The model under review builds one solid part; all positions refer to its coordinate system, in mm. A direction names the side the tool comes from. Coordinates: 2 decimals unless noted, no trailing zeros. Order: outer loops, then holes, each group sorted by start corner. A loop starts at its lowest first (then second) coordinate and runs counter-clockwise, first axis right, second up.
```python
from build123d import *

# Parameters (mm, degrees)
SKETCH2_W                    = 76
SKETCH2_H                    = 120
BASE_FLANGE1_DEPTH           = 1
EDGE_FLANGE1_STRIP_W         = 5.4732
EDGE_FLANGE1_STRIP_H         = 1
EDGE_FLANGE1_STRIP_CUT_DEPTH = 76
EDGE_FLANGE1_DEPTH           = 76
SKETCH10_R                   = 2.063994429
CUT_EXTRUDE1_DEPTH           = 1
SKETCH11_R                   = 5
SKETCH11_R_2                 = 17.5
CUT_EXTRUDE2_DEPTH           = 1


# Sheet-metal steps are written as plain solids
with BuildPart() as part:
    # Sketch2 → Base-Flange1 (new body)
    with BuildSketch(Plane.XY):
        Rectangle(SKETCH2_W, SKETCH2_H)
    extrude(amount=-BASE_FLANGE1_DEPTH)

    # Edge-Flange1 strip (across the edge) → Edge-Flange1 strip cut (cut)
    with BuildSketch(Plane(origin=(38, -60, -1), x_dir=(0, 1, 0), z_dir=(-1, 0, 0))):
        with Locations((-1, -0.5)):
            Rectangle(EDGE_FLANGE1_STRIP_W, EDGE_FLANGE1_STRIP_H)
    extrude(amount=EDGE_FLANGE1_STRIP_CUT_DEPTH, mode=Mode.SUBTRACT)

    # Edge-Flange1 section (across the edge) → Edge-Flange1 (add)
    with BuildSketch(Plane(origin=(38, -60, -1), x_dir=(0, 1, 0), z_dir=(-1, 0, 0))):
        with BuildLine():
            Line((0, 0.7366), (0, 19))
            Line((0, 19), (1, 19))
            Line((1, 19), (1, 0.7366))
            ThreePointArc((1, 0.7366), (1.215745145, 0.215745145), (1.7366, 0))
            Line((1.7366, 0), (1.7366, -1))
            ThreePointArc((1.7366, -1), (0.508638364, -0.491361636), (0, 0.7366))
        make_face()
    extrude(amount=EDGE_FLANGE1_DEPTH)

    # Sketch10 → Cut-Extrude1 (cut)
    with BuildSketch(Plane(origin=(0, -59, 0), x_dir=(1, 0, 0), z_dir=(0, 1, 0))):
        with Locations(Location((-23, 10, 0), (0, 0, 270))):
            Circle(SKETCH10_R)
        with Locations(Location((23, 10, 0), (0, 0, 270))):
            Circle(SKETCH10_R)
    extrude(amount=-CUT_EXTRUDE1_DEPTH, mode=Mode.SUBTRACT)

    # Sketch11 → Cut-Extrude2 (cut)
    with BuildSketch(Plane(origin=(0, 0, -1), x_dir=(-1, 0, 0), z_dir=(0, 0, -1))):
        with Locations((-23.5, -38.2634)):
            Circle(SKETCH11_R)
        with Locations((13, -33.2634)):
            Circle(SKETCH11_R_2)
        with Locations((24.5, -0.7634)):
            Circle(SKETCH11_R)
        with Locations((-23.5, 16.7366)):
            Circle(SKETCH11_R)
    extrude(amount=-CUT_EXTRUDE2_DEPTH, mode=Mode.SUBTRACT)


solid = part.part
```
(1) Draft analysis for pull direction X (two halves, no side actions). For faces 3 (the face through (1, -59, -11)), 4 (the face through (-38, 0.3, -0.4)), 5 (the face through (27.2, 20.1, -0.5)), state which applies: released by +X, released by -X, zero draft, split by the parting line, or undercut.
A:
face 3: zero draft
face 4: released by -X
face 5: undercut
(2) Machinability: for faces 1 (the face through (-25.015, -59.493, -10.447)), 2 (the face through (-1, 2, -1)), which of the approach directions +Z, -Z, +X, -X, +Y, -Y give a long, thin tool a straight path to every point of the face, cutting with its end or side? Answer none if there is none.
A:
face 1: +Y, -Y
face 2: -Z, +X, -X, +Y
(3) Wall thickness on probe 1 along X at (y, z) = (-59.65, -10); probe 2 along Y at (x, z) = (23.5, -0.6); probe 3 along Z at (x, y) = (-20.5, -12.5): over which ranges is each line inside the solid? List them lowest first.
A:
probe 1: x = -38 to -25.06, -20.94 to 20.94, 25.06 to 38
probe 2: y = -59.58 to -43.26, -33.26 to 11.74, 21.74 to 60
probe 3: z = -1 to 0
(4) We need section B-B, the plane z = -10. Write out the cut boundary in (x, y).
A:
outline: (-38, -60) - (-25.06, -60) - (-25.06, -59) - (-38, -59) - close; (-20.94, -60) - (20.94, -60) - (20.94, -59) - (-20.94, -59) - close; (25.06, -60) - (38, -60) - (38, -59) - (25.06, -59) - close
(5) We need section C-C, the plane y = -4.5. Write out the cut boundary in (x, z).
A:
outline: (-38, -1) - (-27.82, -1) - (-27.82, 0) - (-38, 0) - close; (-21.18, -1) - (38, -1) - (38, 0) - (-21.18, 0) - close
(6) For pin 1 Ø16 at (x, y) = (-24.5, -0.76) entering from -Z; pin 2 Ø5.5 at (x, z) = (-23, -10) entering from +Y; pin 3 Ø3.5 at (x, z) = (23, -10) entering from +Y, all flat-tipped, find the tip position at first contact; note any pin that passes through.
A:
pin 1: stops at z = -1
pin 2: stops at y = -59
pin 3: passes through
(7) We need section A-A, the plane x = -13. Write out the cut boundary in (y, z), and give its area (3 significant figures).
A:
outline: (-60, -20) - (-59, -20) - (-59, -1.74) arc R0.74 cw to (-58.26, -1) - (-50.76, -1) - (-50.76, 0) - (-58.26, 0) arc R1.74 ccw to (-60, -1.74) - close; (-15.76, -1) - (60, -1) - (60, 0) - (-15.76, 0) - close
area: 103 mm2
(8) We need section D-D, the plane x = 30. Write out the cut boundary in (y, z).
A:
outline: (-60, -20) - (-59, -20) - (-59, -1.74) arc R0.74 cw to (-58.26, -1) - (60, -1) - (60, 0) - (-58.26, 0) arc R1.74 ccw to (-60, -1.74) - close
